Could you check a few things on this model? Use its own coordinates, in mm. A direction names the side the tool comes from. Give positions to 0.01 mm unless a question says otherwise; leave off trailing zeros. Loops run counter-clockwise (first coordinate to the right, second up) from the corner with the lowest first, then second, coordinate; pieces in that order, holes last. Notation, with made-up numbers: M -36,5 L 22,5 A21 cw 22,21 Z; hole C 10.5,44.25 d11. An arc over 180 degrees is marked long. Return JSON: item names as keys, results as strings. Group by question number.
1. For pin 1 (1 mm diameter, centred on x = -14, z = 14, fed in from +Y); pin 2 (10 mm diameter, centred on x = 16.5, y = -16.5, fed in from +Z), each with a flat end and sliding along its axis, tell me the tip position at first contact or that it passes through.
2. For faces 5 (the flat face through (-21.15, -15, 2)), 6 (the flat face through (5, -11.2, 3)), 7 (the flat face through (13.9, -26, 23)), which set-ups out of +Z, -Z, +X, -X, +Y, -Y let a thin tool reach every point of the face, with its end or its side?
3. If we section it at A-A (z = 17.5): Write out the boundary of the cut face in (x, y), plus the area to 3 significant figures.
4. Please list where these lines run through material, in increasing order: line 1 (Y direction, x = -15.5, z = 2.25); line 2 (X direction, y = -15, z = 1); line 3 (Y direction, x = -15, z = 1).
5. If we section it at B-B (x = 15.5): Write out the boundary of the cut face in (y, z), plus the area to 3 significant figures.
6. If we mould it in two halves opening along X, with no side actions, what happens to faces 1 (the flat face through (-17.1, -26, 22)), 2 (the flat face through (19.6, 19.7, 1.5)), 3 (the flat face through (0, -26, 42)), 4 (the cylindrical face through (14, -15.43, 1.48))? For each: +X half, -X half, draft (parallel to the pull), parting line (faces both ways), or undercut.
7. If we section it at D-D (y = 0): Write out the boundary of the cut face in (x, z).
8. If we section it at C-C (y = -15.5): Write out the boundary of the cut face in (x, z).
```python
from build123d import *

# Parameters (mm, degrees)
SKETCH1_R           = 1.5
SKETCH1_R_2         = 12
BOSS_EXTRUDE1_DEPTH = 3
BOSS_EXTRUDE2_DEPTH = 3
SKETCH3_W           = 42.3
SKETCH3_H           = 3
BOSS_EXTRUDE3_DEPTH = 39
CHAMFER1_SIZE       = 1
CUT_EXTRUDE1_DEPTH  = 3


with BuildPart() as part:
    # Sketch1 → Boss-Extrude1 (new body)
    with BuildSketch(Plane.XY):
        Polygon((-21.15, 18.15), (-18.15, 21.15), (18.15, 21.15), (21.15, 18.15), (21.15, -18.15), (18.15, -21.15), (-18.15, -21.15), (-21.15, -18.15), align=None)
        with Locations((-15.5, 15.5)):
            Circle(SKETCH1_R, mode=Mode.SUBTRACT)
        with Locations((15.5, 15.5)):
            Circle(SKETCH1_R, mode=Mode.SUBTRACT)
        with Locations((15.5, -15.5)):
            Circle(SKETCH1_R, mode=Mode.SUBTRACT)
        with Locations((-15.5, -15.5)):
            Circle(SKETCH1_R, mode=Mode.SUBTRACT)
        Circle(SKETCH1_R_2, mode=Mode.SUBTRACT)
    extrude(amount=BOSS_EXTRUDE1_DEPTH)

    # Sketch2 → Boss-Extrude2 (add)
    with BuildSketch(Plane(origin=(0, 0, 0), x_dir=(-1, 0, 0), z_dir=(0, 0, -1))):
        Polygon((21.15, -18.15), (18.15, -21.15), (-18.15, -21.15), (-21.15, -18.15), (-21.15, -27.15), (21.15, -27.15), align=None)
    extrude(amount=-BOSS_EXTRUDE2_DEPTH)

    # Sketch3 → Boss-Extrude3 (add)
    with BuildSketch(Plane.XY.offset(3)):
        with Locations((0, -25.65)):
            Rectangle(SKETCH3_W, SKETCH3_H)
    extrude(amount=BOSS_EXTRUDE3_DEPTH)

    # Chamfer1
    chamfer1_edges = [part.edges().sort_by_distance(p)[0] for p in [
        (0, -27.15, 0),
    ]]
    chamfer(chamfer1_edges, length=CHAMFER1_SIZE)

    # Sketch4 → Cut-Extrude1 (cut)
    with BuildSketch(Plane(origin=(0, -24.15, 0), x_dir=(1, 0, 0), z_dir=(0, 1, 0))):
        with BuildLine():
            Line((17.1, -7.5), (17.1, -37.5))
            ThreePointArc((17.1, -37.5), (15.5, -39.1), (13.9, -37.5))
            Line((13.9, -37.5), (13.9, -7.5))
            ThreePointArc((13.9, -7.5), (15.5, -5.9), (17.1, -7.5))
        make_face()
        with BuildLine():
            Line((-17.1, -7.5), (-17.1, -37.5))
            ThreePointArc((-17.1, -37.5), (-15.5, -39.1), (-13.9, -37.5))
            Line((-13.9, -37.5), (-13.9, -7.5))
            ThreePointArc((-13.9, -7.5), (-15.5, -5.9), (-17.1, -7.5))
        make_face()
    extrude(amount=-CUT_EXTRUDE1_DEPTH, mode=Mode.SUBTRACT)


solid = part.part
```
Answer:
{
 "1": {"pin 1": "stops at y = -24.15", "pin 2": "stops at z = 3"},
 "2": {"face 5": "+Z, -Z, -X, +Y, -Y", "face 6": "+Z, +X, -X, +Y", "face 7": "+Y, -Y"},
 "3": {"outline": "M -21.15,-27.15 L -17.1,-27.15 L -17.1,-24.15 L -21.15,-24.15 Z; M -13.9,-27.15 L 13.9,-27.15 L 13.9,-24.15 L -13.9,-24.15 Z; M 17.1,-27.15 L 21.15,-27.15 L 21.15,-24.15 L 17.1,-24.15 Z", "area": "108 mm²"},
 "4": {"line 1": "y = -27.15 to -17, -14 to 14, 17 to 21.15", "line 2": "x = -21.15 to -16.91, -14.09 to 14.09, 16.91 to 21.15", "line 3": "y = -27.15 to -16.91, -14.09 to 14.09, 16.91 to 21.15"},
 "5": {"outline": "M -27.15,1 L -26.15,0 L -17,0 L -17,3 L -24.15,3 L -24.15,5.9 L -27.15,5.9 Z; M -27.15,39.1 L -24.15,39.1 L -24.15,42 L -27.15,42 Z; M -14,0 L 14,0 L 14,3 L -14,3 Z; M 17,0 L 21.15,0 L 21.15,3 L 17,3 Z", "area": "144 mm²"},
 "6": {"face 1": "undercut", "face 2": "+X half", "face 3": "draft", "face 4": "undercut"},
 "7": {"outline": "M -21.15,0 L -12,0 L -12,3 L -21.15,3 Z; M 12,0 L 21.15,0 L 21.15,3 L 12,3 Z"},
 "8": {"outline": "M -21.15,0 L -17,0 L -17,3 L -21.15,3 Z; M -14,0 L 14,0 L 14,3 L -14,3 Z; M 17,0 L 21.15,0 L 21.15,3 L 17,3 Z"}
}
